```python
from build123d import *

# Parameters (mm, degrees)
F0_R     = 5.088383
F1_DEPTH = 508
F4_R     = 6.35
F5_DEPTH = 508.001


with BuildPart() as f1:
    # F0 (on Right) → F1 (new body)
    with BuildSketch(Plane.YZ):
        Circle(F0_R)
    extrude(amount=F1_DEPTH)

    # F2 (on Front) → F3 (revolve)
    with BuildSketch(Plane.XZ):
        Polygon((82.693815, 28.264971), (82.693815, 0), (455.550849, 0), (455.550849, 28.264971), (414.656855, 28.264971), (414.656855, 73.970035), (394.209847, 73.970035), (394.209847, 60.739622), (352.113083, 60.739622), (352.113083, 149.744213), (337.679908, 149.744213), (337.679908, 118.47233), (269.122332, 116.066799), (200.564757, 118.47233), (200.564757, 149.744213), (186.131582, 149.744213), (186.131582, 60.739622), (144.034818, 60.739622), (144.034818, 73.970035), (123.58781, 73.970035), (123.58781, 28.264971), align=None)
    revolve(axis=Axis((269.122332, 0, 0), (1, 0, 0)))

    # F4 (on Right) → F5 (cut, through all)
    with BuildSketch(Plane.YZ):
        with Locations((0, 139.7)):
            Circle(F4_R)
        with Locations((0, -139.7)):
            Circle(F4_R)
    extrude(amount=F5_DEPTH, mode=Mode.SUBTRACT)


solid = f1.part
```
Design review of the part built by this model. Coordinates are the model's own, in mm. A direction names the side the tool comes from. Round coordinates to 2 decimals unless told otherwise and drop trailing zeros. Write each loop counter-clockwise with the first axis right and the second up, starting at its lowest first coordinate (ties: lowest second). Pieces come first, ordered by that corner, then holes.
Item 1: We need section B-B on y = -132. Write out the cut boundary in (x, z), and give its area (3 significant figures).
Item 2: The part is to be moulded in two halves that separate along Z. For faces 1 (the conical face through (241.981, 71.204, -92.862)), 2 (the flat face through (352.113, -2, -64)), 3 (the cylindrical face through (344.8, -1.38, 133.5)), say which applies: +Z half, -Z half, draft (parallel to the pull), parting line (faces both ways), or undercut.
Item 3: Clearance check with flat-ended pins moving along their axes: pin 1 Ø16.5 at (y, z) = (0, -139.7) entering from +X; pin 2 Ø5 at (x, y) = (135, 58.5) entering from -Z; pin 3 Ø14.5 at (y, z) = (0, -139.7) entering from -X. State where each tip first meets the part, or that it passes through.
Item 4: For faces 4 (the cylindrical face through (434.818, -28.024, -3.68)), 5 (the cylindrical face through (133.67, 45.01, -58.7)), 6 (the flat face through (186.132, -2, 64)), 7 (the flat face through (508, 0, 0)), list the 3-axis set-ups (+Z, -Z, +X, -X, +Y, -Y) from which the entire face can be reached by the end or side of a thin tool; tool diameter is ignored.
Item 5: For probe 1 along Z at (x, y) = (192, 0); probe 2 along X at (y, z) = (-16.5, 88.5); probe 3 along X at (y, z) = (16.5, 46), list the stretches that pass through material, from the lowest coordinate up.
Item 6: We need section D-D on x = 467.5. Write out the cut boundary in (y, z), and give its area (3 significant figures).
Item 7: We need section C-C on z = -139.7. Write out the cut boundary in (x, y).
Item 8: We need section A-A on z = 125. Write out the cut boundary in (x, y), and give its area (3 significant figures).
Returned:
1. outline: (186.13, -70.71) - (200.56, -70.71) - (200.56, 70.71) - (186.13, 70.71) - close; (337.68, -70.71) - (352.11, -70.71) - (352.11, 70.71) - (337.68, 70.71) - close
1. area: 4,080 mm2
2. face 1: parting line
2. face 2: draft
2. face 3: undercut
3. pin 1: stops at x = 352.11
3. pin 2: stops at z = -48.33
3. pin 3: stops at x = 186.13
4. face 4: +X
4. face 5: -X
4. face 6: none
4. face 7: +Z, -Z, +X, +Y, -Y
5. probe 1: z = -149.74 to -146.05, -133.35 to 133.35, 146.05 to 149.74
5. probe 2: x = 186.13 to 352.11
5. probe 3: x = 123.59 to 414.66
6. outline: circle Ø10.18 at (0, 0)
6. area: 81.3 mm2
7. outline: (186.13, -53.92) - (200.56, -53.92) - (200.56, -6.35) - (186.13, -6.35) - close; (186.13, 6.35) - (200.56, 6.35) - (200.56, 53.92) - (186.13, 53.92) - close; (337.68, -53.92) - (352.11, -53.92) - (352.11, -6.35) - (337.68, -6.35) - close; (337.68, 6.35) - (352.11, 6.35) - (352.11, 53.92) - (337.68, 53.92) - close
8. outline: (186.13, -82.45) - (200.56, -82.45) - (200.56, 82.45) - (186.13, 82.45) - close; (337.68, -82.45) - (352.11, -82.45) - (352.11, 82.45) - (337.68, 82.45) - close
8. area: 4,760 mm2
